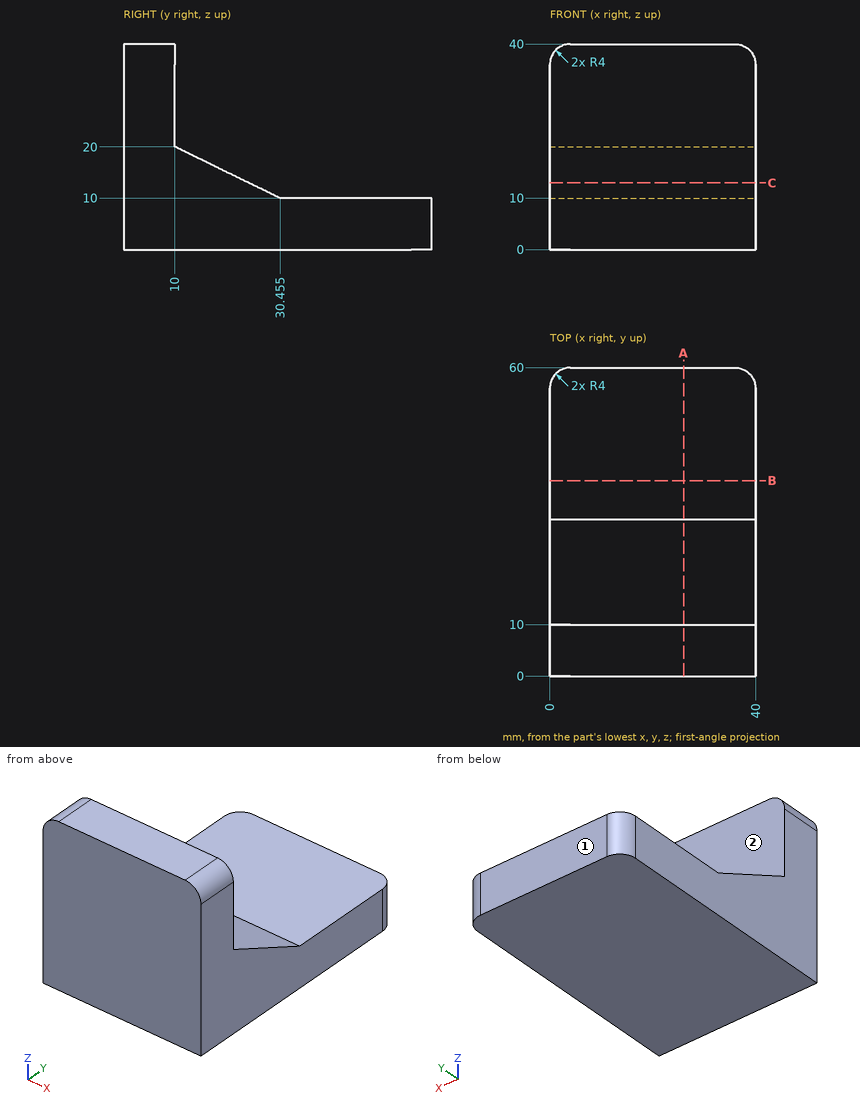
Design review of the part shown in the three views and the two pictorial views. Dimensions are in mm from the part's minimum x, y and z. A direction names the side the tool comes from. Round coordinates to 2 decimals unless told otherwise and drop trailing zeros. Write each loop counter-clockwise with the first axis right and the second up, starting at its lowest first coordinate (ties: lowest second). Pieces come first, ordered by that corner, then holes. Notation, with made-up numbers: (-26.75, 84.25) - (23.25, 84.25) arc R15 cw to (23.25, 97.25) - close; hole circle Ø6 at (18.5, 21.25). An arc over 180 degrees is marked (long way). Write item = value, one per line. Start each with the question number.
1. Wall thickness on L1, parallel to Z at x = 8.5, y = 56; L2, parallel to Y at x = 30, z = 17.5 (1 decimal): over which ranges is each line inside the solid? List them lowest first.
2. For the marked faces 1 and 2, list the 3-axis set-ups (+Z, -Z, +X, -X, +Y, -Y) from which the entire face can be reached by the end or side of a thin tool; tool diameter is ignored.
3. Consider section C-C on z = 13. State the section outline as (x, y) points, plus the area to 3 significant figures.
4. Consider section B-B on y = 38. State the section outline as (x, z) points, plus the area to 3 significant figures.
5. For pin 1 Ø22 at (x, z) = (25, 34.5) entering from +Y; pin 2 Ø10 at (x, z) = (11, 18) entering from +Y; pin 3 Ø15 at (x, y) = (28, 45) entering from +Z, all flat-tipped, find the tip position at first contact; note any pin that passes through.
6. Consider section A-A on x = 26. State the section outline as (y, z) points (1 decimal).
Evaluation:
q1.L1 = 0 to 10
q1.L2 = 0 to 15.1
q2.face_1 = +Z, -Z, +X, -X, +Y
q2.face_2 = +Z, +X, -X, +Y
q3.outline = (0, 0) - (40, 0) - (40, 24.32) - (0, 24.32) - close
q3.area = 973 mm2
q4.outline = (0, 0) - (40, 0) - (40, 10) - (0, 10) - close
q4.area = 400 mm2
q5.pin_1 = 10
q5.pin_2 = 24.32
q5.pin_3 = 10
q6.outline = (0, 0) - (60, 0) - (60, 10) - (30.5, 10) - (10, 20) - (10, 40) - (0, 40) - close
